Input: part model. Units: mm. Frame: model coordinates. Face numbers are marked on the shaded views. A direction names the side the tool comes from. Give positions to 0.01 mm unless a question says otherwise; leave off trailing zeros. Loops run counter-clockwise (first coordinate to the right, second up) from the corner with the lowest first, then second, coordinate; pieces in that order, holes last.
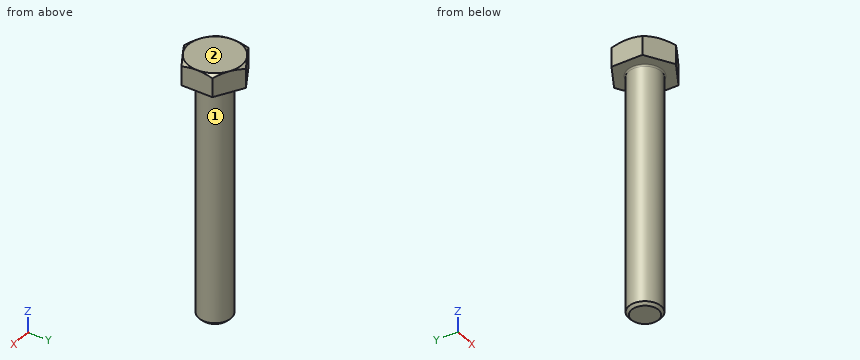
Autodesk Inventor part; units mm, degrees
ref_plane "WorkPlane1" through (0, 0, 0) normal (0, 0, 1) x (1, 0, 0)
ref_plane "MSC_PF1" through (0, 0, 0) normal (1, 0, 0) x (0, 1, 0)
ref_plane "MSC_PT1" through (0, 0, 0) normal (0, 0, -1) x (-1, 0, 0)
ref_plane "WorkPlane1" through (0, 0, 0) normal (0, 0, 1) x (1, 0, 0)
sketch "Sketch1" plane through (0, 0, 0) normal (0, 0, 1) x (1, 0, 0)
  point P0 (0, 0)
sketch "Sketch2" plane through (0, 0, 0) normal (0, 0, 1) x (1, 0, 0)
  line L0 (-5, 2.8868) -> (-5, -2.8868)
  line L1 (0, 5.7734) -> (-5, 2.8868)
  line L2 (5, 2.8868) -> (0, 5.7734)
  line L3 (5, -2.8868) -> (5, 2.8868)
  line L4 (0, -5.7734) -> (5, -2.8868)
  line L5 (-5, -2.8868) -> (0, -5.7734)
  circle A0 centre (0, 0) radius 5 construction
  dimension "d1" = 10
  dimension "d29" = 0
  dimension "d30" = 0
extrude "Extrusion1" add sketch "Sketch2" along normal blind 4
sketch "Sketch3" plane through (0, 0, 0) normal (1, 0, 0) x (0, 1, 0)
  line L0 (5, 4) -> (5.8734, 4)
  line L1 (5.8734, 3.4957) -> (5, 4)
  line L2 (5.8734, 4) -> (5.8734, 3.4957)
  line L3 (0, -0.8) -> (0, 4.8)
  line L4 (5.7734, 0) -> (5.7734, 4)
  dimension "d25" = 0.1
  dimension "d26" = 0
  dimension "d27" = 60
  dimension "d28" = 5
revolve "Revolution1" cut sketch "Sketch3" angle 360 about axis through (0, 0, -10) along (0, 0, 1)
sketch "Sketch4" plane through (0, 0, 0) normal (1, 0, 0) x (0, 1, 0)
  line L0 (0, -45) -> (0, 0)
  line L1 (-3, -45) -> (0, -45)
  line L2 (-3, 0) -> (-3, -45)
  line L3 (0, 0) -> (-3, 0)
  line L4 (0, -45) -> (0, 0)
  line L5 (-3.6, 0) -> (0.6, 0)
  line L6 (0, -54) -> (0, 9)
  dimension "d18" = 3
  dimension "d20" = 45
  dimension "d33" = 0
  dimension "d34" = 0
revolve "Revolution2" add sketch "Sketch4" angle 360 about axis through (0, 0, -45) along (0, 0, -1)
chamfer "Chamfer1" distance 0.5 angle 45 1 edges at (0, 3, -45)
fillet "Fillet1" radius 0.25 1 edges at (0, 3, 0)
thread "Thread1"
ref_plane "MSC_PF1" through (0, 0, 0) normal (1, 0, 0) x (0, 1, 0)
ref_plane "MSC_PT1" through (0, 0, 0) normal (0, 0, -1) x (-1, 0, 0)
equation "\"d22\" = 0.5 * PTC"
equation "\"d23\" = 0.5 * PTC"
equation "\"d24\" = r"
equation "\"d1\" = ParS"
equation "\"d6\" = ParK"
equation "\"d28\" = 0.5 * ParS"
equation "\"d18\" = 0.5 * NND"
equation "\"d20\" = NLG"
equation "\"NND\" = 6"
equation "\"NLG\" = 45"
equation "\"PTC\" = 1"
equation "\"ParK\" = 4"
equation "\"ParS\" = 10"
equation "\"msp_es\" = 0.577367 * ParS"
equation "\"r\" = 0.25"
equation "\"THREADDIA\" = NND"
properties part number "ISO 4016 - M6 x 45" material "Steel"
(1) Ray query, probe 1 along Z at (x, y) = (-3, -2.5); probe 2 along X at (y, z) = (1.75, -14.5); probe 3 along Y at (x, z) = (4.75, 1). Return the intervals inside material, ascending.
Values follow:
probe 1: z = 0 to 4
probe 2: x = -2.44 to 2.44
probe 3: y = -3.03 to 3.03
(2) Pin query (flat end, axial travel): pin 1 Ø4 at (x, z) = (-3, -14) entering from -Y; pin 2 Ø1.5 at (x, y) = (3.5, 3.5) entering from -Z; pin 3 Ø1.5 at (y, z) = (2.5, -29.5) entering from +X. Return the tip coordinate at first contact, or that it passes through.
Values follow:
pin 1: stops at y = -2.83
pin 2: stops at z = 0
pin 3: stops at x = 2.44
(3) Cut plane A-A (z = -8). Return the cut outline in (x, y), and give its area (3 significant figures).
Values follow:
outline: circle Ø6 at (0, 0)
area: 28.3 mm2
(4) Reachability of the marked faces 1 and 2 from +Z, -Z, +X, -X, +Y, -Y: full face, straight path, thin tool, end or side. Return the list, or none.
Values follow:
face 1: -Z
face 2: +Z, +X, -X, +Y, -Y
